```python
from build123d import *

# Parameters (mm, degrees)
SKETCH1_W                      = 20
SKETCH1_H                      = 40
BASE_FLANGE1_DEPTH             = 1.25
EDGE_FLANGE1_STRIP_W           = 7
EDGE_FLANGE1_STRIP_H           = 1.25
EDGE_FLANGE1_STRIP_CUT_DEPTH   = 40
EDGE_FLANGE1_STRIP_2_W         = 7
EDGE_FLANGE1_STRIP_2_H         = 1.25
EDGE_FLANGE1_STRIP_CUT_2_DEPTH = 40
EDGE_FLANGE1_DEPTH             = 40
EDGE_FLANGE1_BEND_DEPTH        = 40
SKETCH12_W                     = 80
SKETCH12_H                     = 50
TAB1_DEPTH                     = 1.25
EDGE_FLANGE2_STRIP_W           = 7
EDGE_FLANGE2_STRIP_H           = 1.25
EDGE_FLANGE2_STRIP_CUT_DEPTH   = 50
EDGE_FLANGE2_STRIP_2_W         = 7
EDGE_FLANGE2_STRIP_2_H         = 1.25
EDGE_FLANGE2_STRIP_CUT_2_DEPTH = 50
EDGE_FLANGE2_DEPTH             = 50
EDGE_FLANGE2_BEND_DEPTH        = 50
EDGE_FLANGE3_DEPTH             = 75.5
TAB2_DEPTH                     = 1.25
SKETCH27_W                     = 6
SKETCH27_H                     = 10
TAB3_DEPTH                     = 1.25
BREAK_CORNER1_START            = 76
BREAK_CORNER1_DEPTH            = 1.25
CUT_EXTRUDE1_REACH             = 102.337
SKETCH30_R                     = 2.5
FILLET1_R                      = 10


# Read off the part's stored shape, not the designer's step: Break-Corner1
# Sheet-metal steps are written as plain solids
with BuildPart() as part:
    # Sketch1 → Base-Flange1 (new body)
    with BuildSketch(Plane(origin=(0, 0, 0), x_dir=(1, 0, 0), z_dir=(0, 1, 0))):
        with Locations((0, 20)):
            Rectangle(SKETCH1_W, SKETCH1_H)
    extrude(amount=-BASE_FLANGE1_DEPTH)

    # Edge-Flange1 strip (across the edge) → Edge-Flange1 strip cut (cut)
    with BuildSketch(Plane(origin=(10, 0, 0), x_dir=(-1, 0, 0), z_dir=(0, 0, -1))):
        with Locations((-1.25, -0.625)):
            Rectangle(EDGE_FLANGE1_STRIP_W, EDGE_FLANGE1_STRIP_H)
    extrude(amount=EDGE_FLANGE1_STRIP_CUT_DEPTH, mode=Mode.SUBTRACT)

    # Edge-Flange1 strip 2 (across the edge) → Edge-Flange1 strip cut 2 (cut)
    with BuildSketch(Plane(origin=(-10, 0, -40), x_dir=(1, 0, 0), z_dir=(0, 0, 1))):
        with Locations((-1.25, -0.625)):
            Rectangle(EDGE_FLANGE1_STRIP_2_W, EDGE_FLANGE1_STRIP_2_H)
    extrude(amount=EDGE_FLANGE1_STRIP_CUT_2_DEPTH, mode=Mode.SUBTRACT)

    # Edge-Flange1 section (across the edge) → Edge-Flange1 (add)
    with BuildSketch(Plane(origin=(10, 0, 0), x_dir=(-1, 0, 0), z_dir=(0, 0, -1))):
        with BuildLine():
            Line((0, 1), (0, 18.75))
            Line((0, 18.75), (1.25, 18.75))
            Line((1.25, 18.75), (1.25, 1))
            ThreePointArc((1.25, 1), (1.542893219, 0.292893219), (2.25, 0))
            Line((2.25, 0), (2.25, -1.25))
            ThreePointArc((2.25, -1.25), (0.659009742, -0.590990258), (0, 1))
        make_face()
    extrude(amount=EDGE_FLANGE1_DEPTH)

    # Edge-Flange1 section 2 (across the edge) → Edge-Flange1 bend (add)
    with BuildSketch(Plane(origin=(-10, 0, -40), x_dir=(1, 0, 0), z_dir=(0, 0, 1))):
        with BuildLine():
            Line((0, 1), (0, 18.75))
            Line((0, 18.75), (1.25, 18.75))
            Line((1.25, 18.75), (1.25, 1))
            ThreePointArc((1.25, 1), (1.542893219, 0.292893219), (2.25, 0))
            Line((2.25, 0), (2.25, -1.25))
            ThreePointArc((2.25, -1.25), (0.659009742, -0.590990258), (0, 1))
        make_face()
    extrude(amount=EDGE_FLANGE1_BEND_DEPTH)

    # Sketch12 → Tab1 (add)
    with BuildSketch(Plane.XZ.offset(1.25)):
        with Locations((0, 25)):
            Rectangle(SKETCH12_W, SKETCH12_H)
    extrude(amount=-TAB1_DEPTH)

    # Edge-Flange2 strip (across the edge) → Edge-Flange2 strip cut (cut)
    with BuildSketch(Plane(origin=(40, 0, 50), x_dir=(-1, 0, 0), z_dir=(0, 0, -1))):
        with Locations((-1.25, -0.625)):
            Rectangle(EDGE_FLANGE2_STRIP_W, EDGE_FLANGE2_STRIP_H)
    extrude(amount=EDGE_FLANGE2_STRIP_CUT_DEPTH, mode=Mode.SUBTRACT)

    # Edge-Flange2 strip 2 (across the edge) → Edge-Flange2 strip cut 2 (cut)
    with BuildSketch(Plane(origin=(-40, 0, 0), x_dir=(1, 0, 0), z_dir=(0, 0, 1))):
        with Locations((-1.25, -0.625)):
            Rectangle(EDGE_FLANGE2_STRIP_2_W, EDGE_FLANGE2_STRIP_2_H)
    extrude(amount=EDGE_FLANGE2_STRIP_CUT_2_DEPTH, mode=Mode.SUBTRACT)

    # Edge-Flange2 section (across the edge) → Edge-Flange2 (add)
    with BuildSketch(Plane(origin=(40, 0, 50), x_dir=(-1, 0, 0), z_dir=(0, 0, -1))):
        with BuildLine():
            Line((0, 1), (0, 30))
            Line((0, 30), (1.25, 30))
            Line((1.25, 30), (1.25, 1))
            ThreePointArc((1.25, 1), (1.542893219, 0.292893219), (2.25, 0))
            Line((2.25, 0), (2.25, -1.25))
            ThreePointArc((2.25, -1.25), (0.659009742, -0.590990258), (0, 1))
        make_face()
    extrude(amount=EDGE_FLANGE2_DEPTH)

    # Edge-Flange2 section 2 (across the edge) → Edge-Flange2 bend (add)
    with BuildSketch(Plane(origin=(-40, 0, 0), x_dir=(1, 0, 0), z_dir=(0, 0, 1))):
        with BuildLine():
            Line((0, 1), (0, 30))
            Line((0, 30), (1.25, 30))
            Line((1.25, 30), (1.25, 1))
            ThreePointArc((1.25, 1), (1.542893219, 0.292893219), (2.25, 0))
            Line((2.25, 0), (2.25, -1.25))
            ThreePointArc((2.25, -1.25), (0.659009742, -0.590990258), (0, 1))
        make_face()
    extrude(amount=EDGE_FLANGE2_BEND_DEPTH)

    # Edge-Flange3 section (across the edge) → Edge-Flange3 (add)
    with BuildSketch(Plane(origin=(-37.75, 0, 76), x_dir=(0, 0, -1), z_dir=(1, 0, 0))):
        with BuildLine():
            Line((-1.25, 26), (-1.25, 30))
            Line((-1.25, 30), (0, 30))
            Line((0, 30), (0, 26))
            ThreePointArc((0, 26), (7.615223689, 7.615223689), (26, 0))
            Line((26, 0), (26, -1.25))
            ThreePointArc((26, -1.25), (6.731340213, 6.731340213), (-1.25, 26))
        make_face()
    extrude(amount=EDGE_FLANGE3_DEPTH)

    # Sketch24 → Tab2 (add)
    with BuildSketch(Plane(origin=(40, 0, 0), x_dir=(0, 0, -1), z_dir=(1, 0, 0))):
        with BuildLine():
            Line((-50, 30), (-77.25, 30))
            Line((-77.25, 30), (-77.25, 26))
            ThreePointArc((-77.25, 26), (-69.120673955, 7.509715389), (-50, 1))
            Line((-50, 1), (-50, 30))
        make_face()
    tab2 = extrude(amount=-TAB2_DEPTH)

    # Mirror1: Tab2 across plane
    add(tab2.mirror(Plane(origin=(0, 0, 0), x_dir=(0, 0, 1), z_dir=(1, 0, 0))))

    # Sketch27 → Tab3 (add)
    with BuildSketch(Plane.XY.offset(77.25)):
        with Locations((-29.75, 35)):
            Rectangle(SKETCH27_W, SKETCH27_H)
        with Locations((-17.85, 35)):
            Rectangle(SKETCH27_W, SKETCH27_H)
        with Locations((-5.95, 35)):
            Rectangle(SKETCH27_W, SKETCH27_H)
        with Locations((5.95, 35)):
            Rectangle(SKETCH27_W, SKETCH27_H)
        with Locations((17.85, 35)):
            Rectangle(SKETCH27_W, SKETCH27_H)
        with Locations((29.75, 35)):
            Rectangle(SKETCH27_W, SKETCH27_H)
    extrude(amount=-TAB3_DEPTH)

    # Break-Corner1 outline → Break-Corner1 (cut)
    with BuildSketch(Plane.XY.offset(BREAK_CORNER1_START)):
        Polygon((-37.75, 30), (-37.75, 27), (-34.75, 30), align=None)
        Polygon((-26.75, 40), (-29.75, 40), (-26.75, 37), align=None)
        Polygon((-32.75, 40), (-32.75, 37), (-29.75, 40), align=None)
        Polygon((-20.85, 40), (-20.85, 37), (-17.85, 40), align=None)
        Polygon((-14.85, 40), (-17.85, 40), (-14.85, 37), align=None)
        Polygon((-8.95, 40), (-8.95, 37), (-5.95, 40), align=None)
        Polygon((-2.95, 40), (-5.95, 40), (-2.95, 37), align=None)
        Polygon((2.95, 40), (2.95, 37), (5.95, 40), align=None)
        Polygon((8.95, 40), (5.95, 40), (8.95, 37), align=None)
        Polygon((14.85, 40), (14.85, 37), (17.85, 40), align=None)
        Polygon((20.85, 40), (17.85, 40), (20.85, 37), align=None)
        Polygon((26.75, 40), (26.75, 37), (29.75, 40), align=None)
        Polygon((37.75, 30), (34.75, 30), (37.75, 27), align=None)
        Polygon((32.75, 40), (29.75, 40), (32.75, 37), align=None)
    extrude(amount=BREAK_CORNER1_DEPTH, mode=Mode.SUBTRACT)

    # Cut-Extrude1: up to this face of the body (flat: up to its plane)
    cut_extrude1_end = Plane(part.part.faces().sort_by_distance((-10, 9.875, -20))[0])
    # Sketch30 → Cut-Extrude1 (cut, up to the picked face)
    with BuildSketch(Plane(origin=(10, 0, 0), x_dir=(0, 0, -1), z_dir=(1, 0, 0)), mode=Mode.PRIVATE) as cut_extrude1_sk1:
        with Locations(Location((32.5, 6.25, 0), (0, 0, 90))):
            Circle(SKETCH30_R)
    cut_extrude1_tool1 = split(extrude(cut_extrude1_sk1.sketch, amount=-CUT_EXTRUDE1_REACH, mode=Mode.PRIVATE), bisect_by=cut_extrude1_end, keep=Keep.BOTH, mode=Mode.PRIVATE)
    add(cut_extrude1_tool1.solids().sort_by(Axis((10, 6.25, -32.5), (-1, 0, 0)))[0], mode=Mode.SUBTRACT)

    # Fillet1
    fillet1_edges = [part.edges().sort_by_distance(p)[0] for p in [
        (9.375, 18.75, -40),
        (-9.375, 18.75, -40),
    ]]
    fillet(fillet1_edges, radius=FILLET1_R)


solid = part.part
```
CAD build for the part. Positions are in the model's coordinates, mm. A direction names the side the tool comes from. Give positions to 0.01 mm unless a question says otherwise; leave off trailing zeros. Loops run counter-clockwise (first coordinate to the right, second up) from the corner with the lowest first, then second, coordinate; pieces in that order, holes last. Notation, with made-up numbers: (34, 46) - (58, 46) arc R22 cw to (58, 84) - close; hole circle Ø11 at (-27, 89.5). An arc over 180 degrees is marked (long way). Put each result on its own line as item: value.
Q1. Mould opens along X. For faces 1 (the face through (-9.32, -0.61, -20.28)), 2 (the face through (-39.384, 7.708, 69.334)), 3 (the face through (-7.47, 38.48, 76.62)) say: pulls with the +X half, pulls with the -X half, needs draft (parallel to the pull), parting line crosses it, or undercut.
Filled in:
face 1: pulls with the -X half
face 2: needs draft
face 3: undercut
Q2. Slice it at A-A (z = 58.5). Give the cut face in (x, y), plus the area to 3 significant figures.
Filled in:
outline: (-40, 1.72) - (-38.75, 1.72) - (-38.75, 30) - (-40, 30) - close; (-37.75, 0.11) - (37.75, 0.11) - (37.75, 1.43) - (-37.75, 1.43) - close; (38.75, 1.72) - (40, 1.72) - (40, 30) - (38.75, 30) - close
area: 170 mm²
Q3. Probe line 1 along X through (y, z) = (22, 63); line 2 along Z through (x, y) = (9, 6); line 3 along Z through (x, y) = (-9.55, 6.25). List the from-to ranges inside material, lowest first.
Filled in:
line 1: x = -40 to -38.75, 38.75 to 40
line 2: z = -40 to -34.99, -30.01 to 0, 66.61 to 68.51
line 3: z = -40 to -35, -30 to 0, 66.91 to 68.77
Q4. Slice it at C-C (x = 31). Give the cut face in (y, z).
Filled in:
outline: (-1.25, 0) - (0, 0) - (0, 50) arc R26 cw to (26, 76) - (38.75, 76) - (38.75, 77.25) - (26, 77.25) arc R27.25 ccw to (-1.25, 50) - close
Q5. Flat gauge pins, fed straight in: pin 1 (1.4 mm diameter, centred on x = 0, z = 76.5, fed in from +Y); pin 2 (10 mm diameter, centred on x = 23.5, y = 31, fed in from -Z); pin 3 (0.6 mm diameter, centred on y = 34.5, z = 77, fed in from +X); pin 4 (4 mm diameter, centred on y = 6.25, z = -32.5, fed in from -X). Where does each tip first touch, or does it go through?
Filled in:
pin 1: stops at y = 30
pin 2: stops at z = 76
pin 3: stops at x = 32.75
pin 4: passes through
Q6. Slice it at D-D (y = 21). Give the cut face in (x, z), plus the area to 3 significant figures.
Filled in:
outline: (-40, 0) - (-38.75, 0) - (-38.75, 76.75) - (-40, 76.75) - close; (-37.75, 75.51) - (37.75, 75.51) - (37.75, 76.79) - (-37.75, 76.79) - close; (38.75, 0) - (40, 0) - (40, 76.75) - (38.75, 76.75) - close
area: 288 mm²
Q7. Tool access for faces 4 (the face through (-0.5, 29.8, 77.25)), 5 (the face through (-16.37, 38.52, 76.62)): list every direction of +Z, -Z, +X, -X, +Y, -Y with a clear straight run to the whole face (end or side of a thin tool).
Filled in:
face 4: +Z, +X, -X, +Y, -Y
face 5: +Z, -Z, +Y
Q8. Slice it at B-B (y = 12.5). Give the cut face in (x, z), plus the area to 3 significant figures.
Filled in:
outline: (-40, 0) - (-38.75, 0) - (-38.75, 73.31) - (-40, 73.31) - close; (-37.75, 72.22) - (37.75, 72.22) - (37.75, 73.67) - (-37.75, 73.67) - close; (-10, -39.27) - (-8.75, -39.27) - (-8.75, 0) - (-10, 0) - close; (8.75, -39.27) - (10, -39.27) - (10, 0) - (8.75, 0) - close; (38.75, 0) - (40, 0) - (40, 73.31) - (38.75, 73.31) - close
area: 391 mm²
